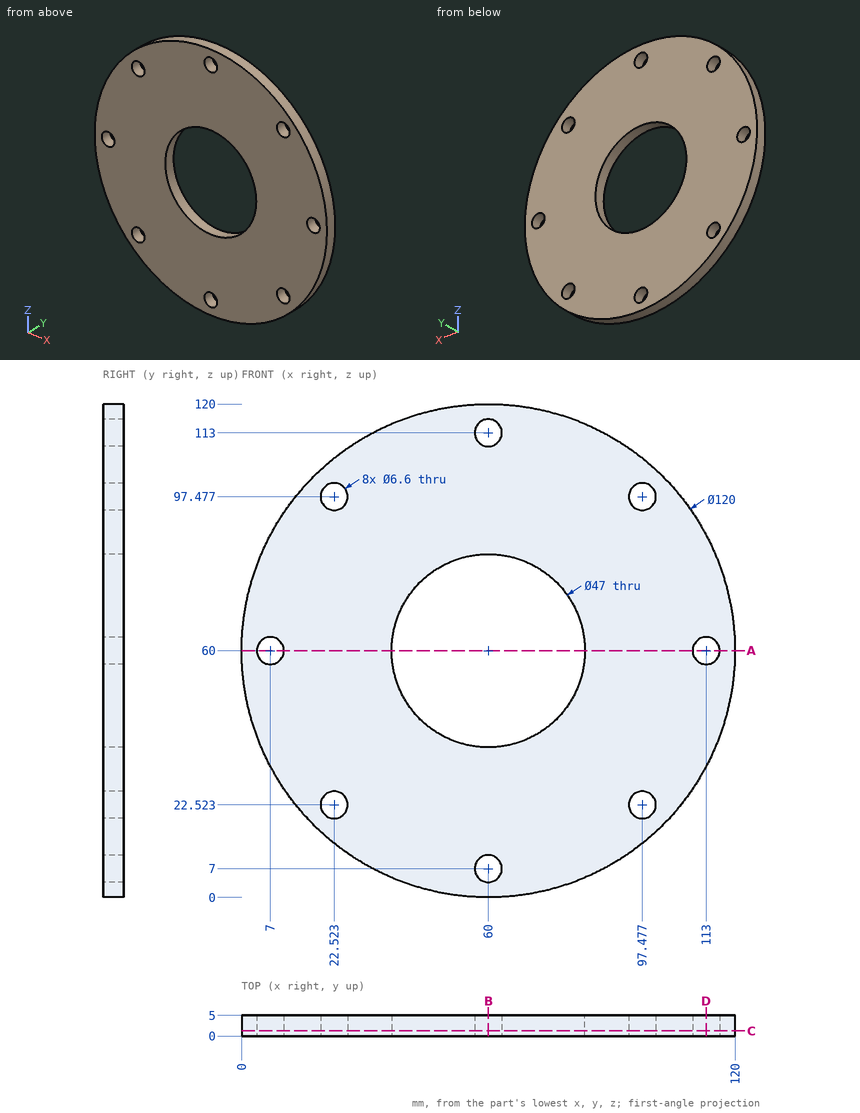
Geometry check sheet. Reference: drawing and pictorial views, mm from the part's lowest x, y, z. Give positions to 0.01 mm unless a question says otherwise; leave off trailing zeros. Write each loop counter-clockwise with the first axis right and the second up, starting at its lowest first coordinate (ties: lowest second). Pieces come first, ordered by that corner, then holes. Notation, with made-up numbers: M 7,82 L 52,82 A21 ccw 52,104 Z; hole C -25.75,66.5 d6. An arc over 180 degrees is marked long. Put each result on its own line as item: value. Start each with the question number.
1. Go/stop test with flat-tipped pins: pin 1 Ø3 at (y, z) = (2.5, 54) entering from +X; pin 2 Ø2 at (y, z) = (2.5, 97.5) entering from -X; pin 3 Ø1 at (y, z) = (1, 52) entering from -X. Record where each tip stops, or that it passes through.
2. Section check B-B (x = 60). Record the cut outline in (y, z), and give its area (3 significant figures).
3. Scan lines: line 1 along X through (y, z) = (2, 60); line 2 along Z through (x, y) = (7, 3.6) (1 decimal). Record each from-to range of solid material in increasing order. Write a range as [from, to].
4. Section check D-D (x = 113). Record the cut outline in (y, z) (1 decimal).
5. Section check A-A (z = 60). Record the cut outline in (x, y), and give its area (3 significant figures).
6. Section check C-C (y = 1.25). Give the number of separate pieces and of enclosed holes in the cut face, and give its area (3 significant figures).
Answer list:
1. pin 1: x = 119.83
1. pin 2: x = 12.38
1. pin 3: x = 0.47
2. outline: M 0,0 L 5,0 L 5,3.7 L 0,3.7 Z; M 0,10.3 L 5,10.3 L 5,36.5 L 0,36.5 Z; M 0,83.5 L 5,83.5 L 5,109.7 L 0,109.7 Z; M 0,116.3 L 5,116.3 L 5,120 L 0,120 Z
2. area: 299 mm2
3. line 1: [0, 3.7], [10.3, 36.5], [83.5, 109.7], [116.3, 120]
3. line 2: [31.9, 56.7], [63.3, 88.1]
4. outline: M 0,31.9 L 5,31.9 L 5,56.7 L 0,56.7 Z; M 0,63.3 L 5,63.3 L 5,88.1 L 0,88.1 Z
5. outline: M 0,0 L 3.7,0 L 3.7,5 L 0,5 Z; M 10.3,0 L 36.5,0 L 36.5,5 L 10.3,5 Z; M 83.5,0 L 109.7,0 L 109.7,5 L 83.5,5 Z; M 116.3,0 L 120,0 L 120,5 L 116.3,5 Z
5. area: 299 mm2
6. separate pieces: 1
6. enclosed holes: 9
6. area: 9,300 mm2
